Check sheet for the drawn part. Datum: minimum x, y, z corner. Units: mm. Coordinates: 2 decimals unless noted, no trailing zeros. Loops run counter-clockwise (first coordinate to the right, second up) from the corner with the lowest first, then second, coordinate; pieces in that order, holes last. Notation, with made-up numbers: M 5.25,7.25 L 31.25,7.25 A23 cw 31.25,19.25 Z; hole C 25,-28 d5. An arc over 180 degrees is marked long. Use CSV: the item, a comma, the result in double quotes. Start each with the question number.
(1) Section check A-A on y = 13.5. Record the cut outline in (x, z).
(2) Go/stop test with flat-tipped pins: pin 1 Ø10 at (y, z) = (18.5, 23) entering from -X; pin 2 Ø4 at (y, z) = (32, 68.5) entering from +X; pin 3 Ø1.5 at (y, z) = (24, 35) entering from +X. Record where each tip stops, or that it passes through.
(3) Scan lines: line 1 (Y direction, x = 29, z = 87); line 2 (X direction, y = 5, z = 89); line 3 (X direction, y = 35, z = 51). Record each from-to range of solid material in increasing order.
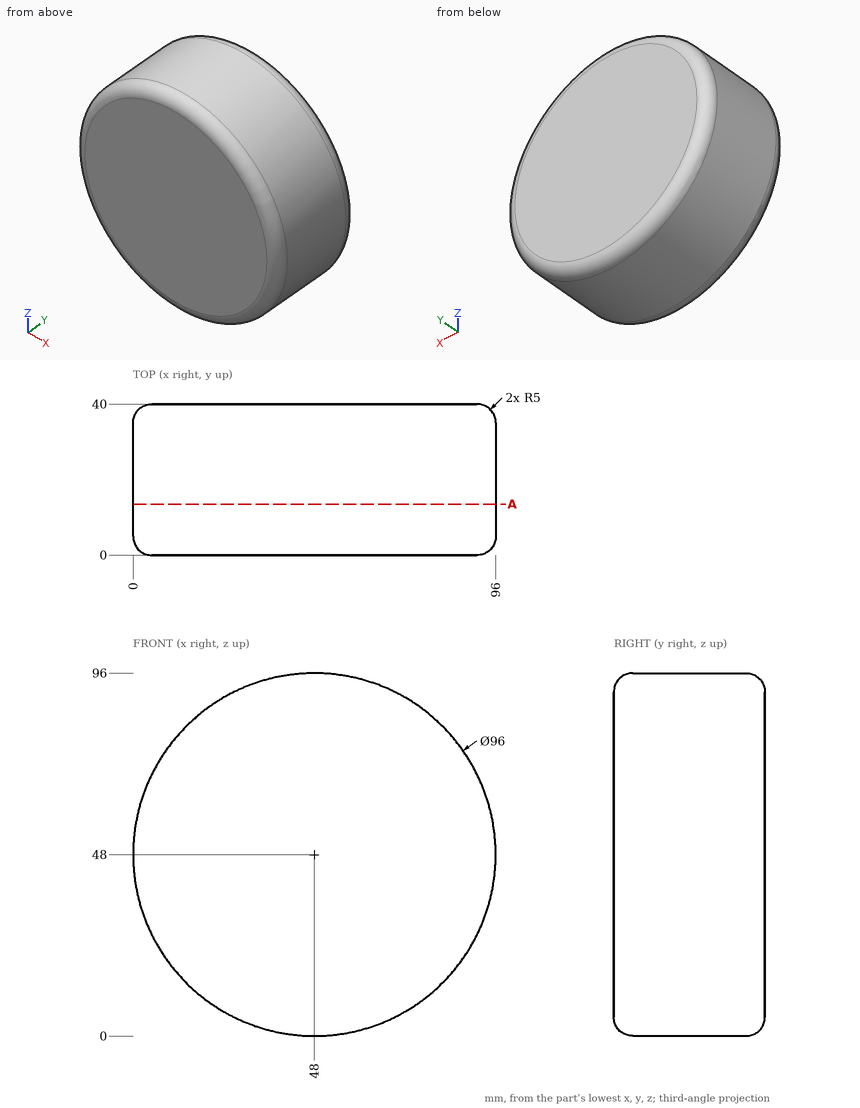
Outcome:
1,outline,"C 48,48 d96"
2,pin 1,"stops at x = 4.37"
2,pin 2,"stops at x = 92.29"
2,pin 3,"stops at x = 94.41"
3,line 1,"y = 0.01 to 39.99"
3,line 2,"x = 23.04 to 72.96"
3,line 3,"x = 0.09 to 95.91"
